Geometry check sheet. Reference: drawing and pictorial views, mm from the part's lowest x, y, z. A direction names the side the tool comes from. Round coordinates to 2 decimals unless told otherwise and drop trailing zeros. Loops run counter-clockwise (first coordinate to the right, second up) from the corner with the lowest first, then second, coordinate; pieces in that order, holes last. Notation, with made-up numbers: (-13.5, 88.5) - (17.5, 88.5) arc R11 cw to (17.5, 101.5) - close; hole circle Ø9 at (10.25, 84.25). An arc over 180 degrees is marked (long way). Return JSON: item names as keys, results as strings.
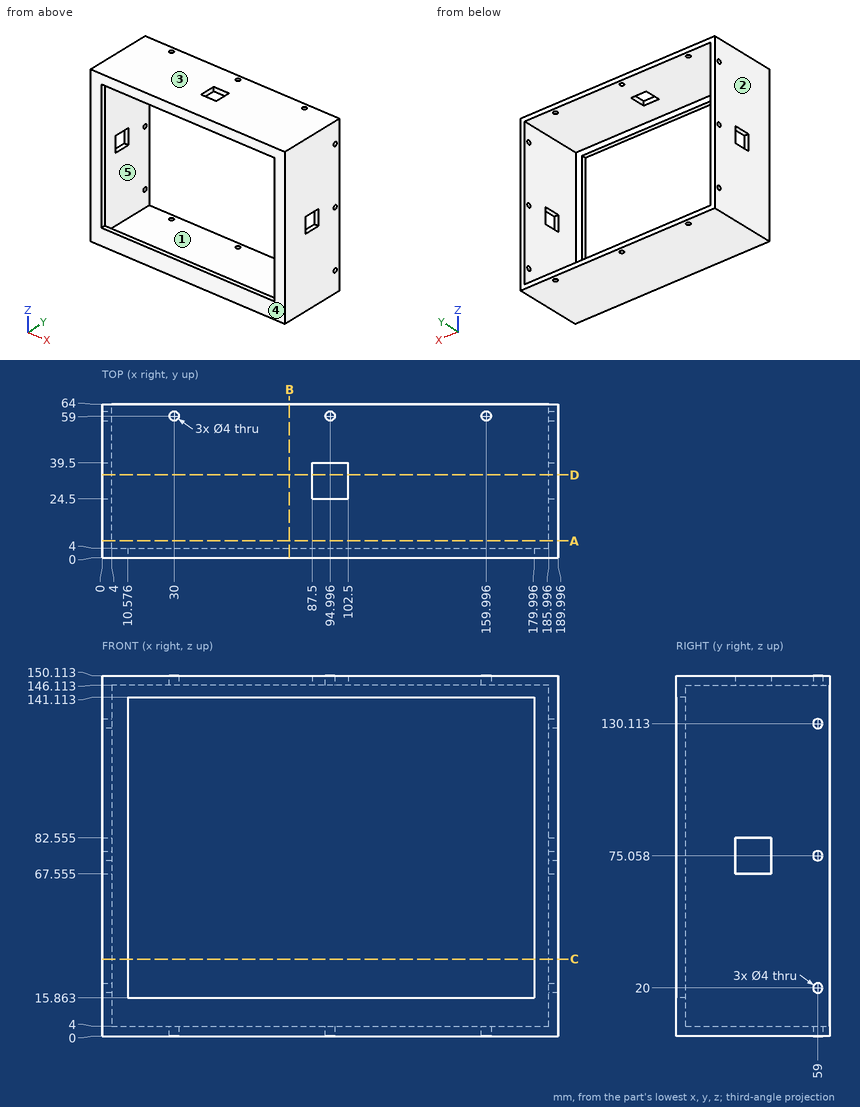
Q1. Sectioned sample at D-D (y = 34.5). Enter the section's corners in (x, z) (1 decimal), plus the area to 3 significant figures.
Answer key:
{"outline": "(0, 0) - (190, 0) - (190, 67.6) - (186, 67.6) - (186, 4) - (4, 4) - (4, 67.6) - (0, 67.6) - close; (0, 82.6) - (4, 82.6) - (4, 146.1) - (87.5, 146.1) - (87.5, 150.1) - (0, 150.1) - close; (102.5, 146.1) - (186, 146.1) - (186, 82.6) - (190, 82.6) - (190, 150.1) - (102.5, 150.1) - close", "area": "2,480 mm²"}
Q2. Tool access check on the marked faces 1 and 2. Record the directions out of +Z, -Z, +X, -X, +Y, -Y that give a thin tool (end or side, any length) a straight path to the whole face; none if there is none.
Answer key:
{"face 1": "+Y", "face 2": "+Z, -Z, -X, +Y, -Y"}
Q3. Depth check by flat-ended pin: P1, Ø12, axis at x = 27.5, z = 26, coming from the -Y side (3 decimals). Enter the tip coordinate at first touch or a pass-through.
Answer key:
{"P1": "passes through"}
Q4. Sectioned sample at A-A (y = 7). Enter the section's corners in (x, z).
Answer key:
{"outline": "(0, 0) - (190, 0) - (190, 150.11) - (0, 150.11) - close; hole (4, 4) - (186, 4) - (186, 146.11) - (4, 146.11) - close"}
Q5. Scan lines: probe 1 along X at (y, z) = (12, 123.5); probe 2 along Z at (x, y) = (35, 38); probe 3 along Y at (x, z) = (104.5, 11). Record each from-to range of solid material in increasing order. Write a range as [from, to].
Answer key:
{"probe 1": "x = [0, 4], [186, 190]", "probe 2": "z = [0, 4], [146.11, 150.11]", "probe 3": "y = [0, 4]"}
Q6. Sectioned sample at C-C (z = 32). Enter the section's corners in (x, y).
Answer key:
{"outline": "(0, 0) - (10.58, 0) - (10.58, 4) - (4, 4) - (4, 64) - (0, 64) - close; (180, 0) - (190, 0) - (190, 64) - (186, 64) - (186, 4) - (180, 4) - close"}
Q7. Sectioned sample at B-B (x = 78). Enter the section's corners in (y, z).
Answer key:
{"outline": "(0, 0) - (64, 0) - (64, 4) - (4, 4) - (4, 15.86) - (0, 15.86) - close; (0, 141.11) - (4, 141.11) - (4, 146.11) - (64, 146.11) - (64, 150.11) - (0, 150.11) - close"}
Q8. Draft check along Z on the marked faces 3, 4 and 5. Enter one of: released by +Z, released by -Z, zero draft, split by the parting line, or undercut.
Answer key:
{"face 3": "released by +Z", "face 4": "zero draft", "face 5": "undercut"}
